Check sheet for the drawn part. Datum: minimum x, y, z corner. Units: mm. A direction names the side the tool comes from. Give positions to 0.01 mm unless a question says otherwise; leave off trailing zeros. Write each loop counter-clockwise with the first axis right and the second up, starting at its lowest first coordinate (ties: lowest second). Pieces come first, ordered by that corner, then holes.
(1) Cross-section at D-D (z = 43.5). Record the boundary of the cut face in (x, y).
(2) Cross-section at C-C (y = 16.5). Record the boundary of the cut face in (x, z).
(3) Cross-section at B-B (x = 142.5). Record the boundary of the cut face in (y, z), and give its area (4 significant figures).
(4) Cross-section at A-A (y = 52). Record the boundary of the cut face in (x, z).
(5) Thickness scan on line 1 along X through (y, z) = (8.5, 96); line 2 along Z through (x, y) = (80, 51); line 3 along Y through (x, z) = (121, 55.5). Record the ranges inside material, lowest first.
(6) Mould release check, pull along X, two halves, no side actions. Record for the marked faces 3, 4, 5 and 6: +X half, -X half, draft (parallel to the pull), parting line (faces both ways), or undercut.
(7) Tool access check on the marked faces 1 and 2. Record the directions out of +Z, -Z, +X, -X, +Y, -Y that give a thin tool (end or side, any length) a straight path to the whole face; none if there is none.
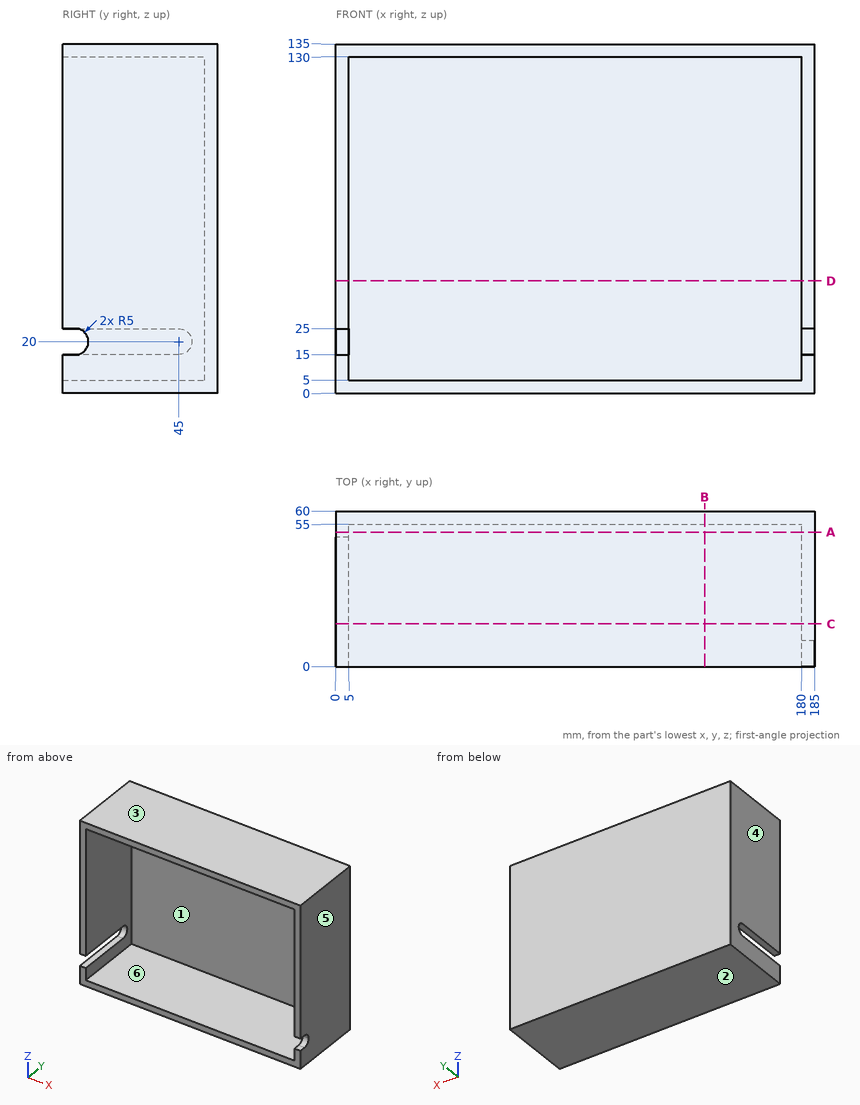
Reply:
1. outline: (0, 0) - (5, 0) - (5, 55) - (180, 55) - (180, 0) - (185, 0) - (185, 60) - (0, 60) - close
2. outline: (0, 0) - (185, 0) - (185, 135) - (0, 135) - (0, 25) - (5, 25) - (5, 130) - (180, 130) - (180, 5) - (5, 5) - (5, 15) - (0, 15) - close
3. outline: (0, 0) - (60, 0) - (60, 135) - (0, 135) - (0, 130) - (55, 130) - (55, 5) - (0, 5) - close
3. area: 1,225 mm2
4. outline: (0, 0) - (185, 0) - (185, 135) - (0, 135) - close; hole (5, 5) - (180, 5) - (180, 130) - (5, 130) - close
5. line 1: x = 0 to 5, 180 to 185
5. line 2: z = 0 to 5, 130 to 135
5. line 3: y = 55 to 60
6. face 3: draft
6. face 4: -X half
6. face 5: +X half
6. face 6: undercut
7. face 1: -Y
7. face 2: -Z, +X, -X, +Y, -Y
